Read the model definition and answer for the solid it produces. Units are mm, in the model's axes. Coordinates: 2 decimals unless noted, no trailing zeros. Order: outer loops, then holes, each group sorted by start corner. A loop starts at its lowest first (then second) coordinate and runs counter-clockwise, first axis right, second up.
```python
from build123d import *

# Parameters (mm, degrees)
ESQUISSE1_W             = 185
ESQUISSE1_H             = 9
ESQUISSE1_R             = 2
BOSS_EXTRU_1_DEPTH      = 7
ENL_V_MAT_EXTRU_1_REACH = 187
ESQUISSE2_W             = 2
ESQUISSE2_H             = 2
CHANFREIN1_SIZE         = 1


with BuildPart() as part:
    # Esquisse1 → Boss.-Extru.1 (new body)
    with BuildSketch(Plane.XY):
        Rectangle(ESQUISSE1_W, ESQUISSE1_H)
        with Locations((-80, 0)):
            Circle(ESQUISSE1_R, mode=Mode.SUBTRACT)
        with Locations((-60, 0)):
            Circle(ESQUISSE1_R, mode=Mode.SUBTRACT)
        with Locations((-40, 0)):
            Circle(ESQUISSE1_R, mode=Mode.SUBTRACT)
        with Locations((-20, 0)):
            Circle(ESQUISSE1_R, mode=Mode.SUBTRACT)
        Circle(ESQUISSE1_R, mode=Mode.SUBTRACT)
        with Locations((20, 0)):
            Circle(ESQUISSE1_R, mode=Mode.SUBTRACT)
        with Locations((40, 0)):
            Circle(ESQUISSE1_R, mode=Mode.SUBTRACT)
        with Locations((60, 0)):
            Circle(ESQUISSE1_R, mode=Mode.SUBTRACT)
        with Locations((80, 0)):
            Circle(ESQUISSE1_R, mode=Mode.SUBTRACT)
    extrude(amount=BOSS_EXTRU_1_DEPTH)

    # Esquisse2 → Enlèv. mat.-Extru.1 (cut, up to next)
    with BuildSketch(Plane.ZY.offset(92.5), mode=Mode.PRIVATE) as enl_v_mat_extru_1_sk1:
        with Locations((2, 3.5)):
            Rectangle(ESQUISSE2_W, ESQUISSE2_H)
    enl_v_mat_extru_1_tool1 = extrude(enl_v_mat_extru_1_sk1.sketch, amount=-ENL_V_MAT_EXTRU_1_REACH, mode=Mode.PRIVATE) & part.part
    add(enl_v_mat_extru_1_tool1.solids().sort_by_distance((-92.5, 3.5, 2))[0], mode=Mode.SUBTRACT)
    # Esquisse2 → Enlèv. mat.-Extru.1 (cut, up to next)
    with BuildSketch(Plane.ZY.offset(92.5), mode=Mode.PRIVATE) as enl_v_mat_extru_1_sk2:
        with Locations((2, -3.5)):
            Rectangle(ESQUISSE2_W, ESQUISSE2_H)
    enl_v_mat_extru_1_tool2 = extrude(enl_v_mat_extru_1_sk2.sketch, amount=-ENL_V_MAT_EXTRU_1_REACH, mode=Mode.PRIVATE) & part.part
    add(enl_v_mat_extru_1_tool2.solids().sort_by_distance((-92.5, -3.5, 2))[0], mode=Mode.SUBTRACT)

    # Chanfrein1
    chanfrein1_edges = [part.edges().sort_by_distance(p)[0] for p in [
        (-82, 0, 7),
        (-62, 0, 7),
        (-42, 0, 7),
        (-22, 0, 7),
        (-2, 0, 7),
        (18, 0, 7),
        (38, 0, 7),
        (58, 0, 7),
        (78, 0, 7),
    ]]
    chamfer(chanfrein1_edges, length=CHANFREIN1_SIZE)


solid = part.part
```
1) A flat-ended cylindrical pin translates along its axis: pin 1 Ø4.5 at (x, y) = (-60, 0) entering from +Z. Find the tip coordinate at first contact, or state that the pin passes through.
A:
pin 1: stops at z = 6.25
2) A cutting plane is placed at A-A, the plane x = 0. Determine the outline of the cut face in (y, z), and give its area (3 significant figures).
A:
outline: (-4.5, 0) - (-2, 0) - (-2, 6) - (-3, 7) - (-4.5, 7) - (-4.5, 3) - (-2.5, 3) - (-2.5, 1) - (-4.5, 1) - close; (2, 0) - (4.5, 0) - (4.5, 1) - (2.5, 1) - (2.5, 3) - (4.5, 3) - (4.5, 7) - (3, 7) - (2, 6) - close
area: 26.0 mm2
3) Straight lines are drawn through the part: line 1 (Z direction, x = -65.5, y = -3); line 2 (Y direction, x = 0, z = 4.35); line 3 (Y direction, x = -60, z = 2). For each, find the intervals that lie inside material, in ascending order.
A:
line 1: z = 0 to 1, 3 to 7
line 2: y = -4.5 to -2, 2 to 4.5
line 3: y = -2.5 to -2, 2 to 2.5
4) A cutting plane is placed at B-B, the plane y = 0. State how many separate pieces and enclosed holes the cut face has, and give its area (3 significant figures).
A:
separate pieces: 10
enclosed holes: 0
area: 1,030 mm2
5) Determine the mould class of faces 1 (the flat face through (92.5, 0, 3)), 2 (the cylindrical face through (-42, 0, 3)), 3 (the flat face through (-1, -4.5, 5)) for opening direction Y: pulls with the +Y half, pulls with the -Y half, needs draft (parallel to the pull), parting line crosses it, or undercut.
A:
face 1: needs draft
face 2: undercut
face 3: pulls with the -Y half
6) A cutting plane is placed at C-C, the plane x = -72. Determine the outline of the cut face in (y, z), and give its area (3 significant figures).
A:
outline: (-4.5, 0) - (4.5, 0) - (4.5, 1) - (2.5, 1) - (2.5, 3) - (4.5, 3) - (4.5, 7) - (-4.5, 7) - (-4.5, 3) - (-2.5, 3) - (-2.5, 1) - (-4.5, 1) - close
area: 55.0 mm2
